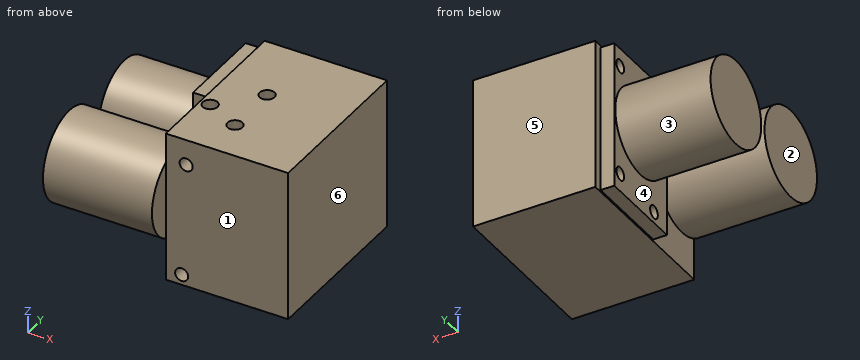
```python
from build123d import *

# Parameters (mm, degrees)
SKETCH2_W                        = 98.18
SKETCH2_H                        = 135.15
BOSS_EXTRUDE1_DEPTH              = 55.6
BOSS_EXTRUDE1_DEPTH_BACK         = 65.6
SKETCH3_R                        = 34.65
SKETCH3_R_2                      = 35.85
BOSS_EXTRUDE2_DEPTH              = 87.5
TAP_DRILL_FOR_M14X2_0_TAP1_D     = 12
TAP_DRILL_FOR_M14X2_0_TAP1_DEPTH = 19.56
TAP_DRILL_FOR_M14X2_0_TAP1_TIP   = 3.605163714
TAP_DRILL_FOR_M12X1_5_TAP2_D     = 10.5
TAP_DRILL_FOR_M12X1_5_TAP2_DEPTH = 19.56
TAP_DRILL_FOR_M12X1_5_TAP2_TIP   = 3.15451825
SKETCH8_W                        = 118.2
SKETCH8_H                        = 72
BOSS_EXTRUDE3_DEPTH              = 11
TAP_DRILL_FOR_M12X1_5_TAP3_D     = 10.5
TAP_DRILL_FOR_M12X1_5_TAP3_DEPTH = 19.56
TAP_DRILL_FOR_M12X1_5_TAP3_TIP   = 3.15451825


with BuildPart() as part:
    # Sketch2 → Boss-Extrude1 (new body, two sides)
    with BuildSketch(Plane.XY) as boss_extrude1_sk:
        Rectangle(SKETCH2_W, SKETCH2_H)
    extrude(amount=BOSS_EXTRUDE1_DEPTH)
    extrude(boss_extrude1_sk.sketch, amount=-BOSS_EXTRUDE1_DEPTH_BACK)

    # Sketch3 → Boss-Extrude2 (add)
    with BuildSketch(Plane.ZY.offset(49.09)):
        with Locations((0, 24.325)):
            Circle(SKETCH3_R)
        with Locations((0, -50.675)):
            Circle(SKETCH3_R_2)
    extrude(amount=BOSS_EXTRUDE2_DEPTH)

    # Tap Drill for M14x2.0 Tap1
    with Locations(Plane.XY.offset(55.6)):
        with Locations((-13.23, 9.825), (-13.23, -34.075), (-41.09, -20.575)):
            Hole(TAP_DRILL_FOR_M14X2_0_TAP1_D / 2, depth=TAP_DRILL_FOR_M14X2_0_TAP1_DEPTH)
            with Locations((0, 0, -(TAP_DRILL_FOR_M14X2_0_TAP1_DEPTH + TAP_DRILL_FOR_M14X2_0_TAP1_TIP / 2))):  # 118° drill point
                Cone(0, TAP_DRILL_FOR_M14X2_0_TAP1_D / 2, TAP_DRILL_FOR_M14X2_0_TAP1_TIP, mode=Mode.SUBTRACT)

    # Tap Drill for M12x1.5 Tap2
    with Locations(Plane(origin=(0, -67.575, 0), x_dir=(-1, 0, 0), z_dir=(0, -1, 0))):
        with Locations((32.79, -35.1), (36.39, 57.2)):
            Hole(TAP_DRILL_FOR_M12X1_5_TAP2_D / 2, depth=TAP_DRILL_FOR_M12X1_5_TAP2_DEPTH)
            with Locations((0, 0, -(TAP_DRILL_FOR_M12X1_5_TAP2_DEPTH + TAP_DRILL_FOR_M12X1_5_TAP2_TIP / 2))):  # 118° drill point
                Cone(0, TAP_DRILL_FOR_M12X1_5_TAP2_D / 2, TAP_DRILL_FOR_M12X1_5_TAP2_TIP, mode=Mode.SUBTRACT)

    # Sketch8 → Boss-Extrude3 (add)
    with BuildSketch(Plane.ZY.offset(49.09)):
        with Locations((-5, 24.325)):
            Rectangle(SKETCH8_W, SKETCH8_H)
    extrude(amount=BOSS_EXTRUDE3_DEPTH)

    # Tap Drill for M12x1.5 Tap3
    with Locations(Plane.ZY.offset(60.09)):
        with Locations((-49.6, 52.175), (-55.1, 6.075), (45.1, 6.075), (39.6, 52.175)):
            Hole(TAP_DRILL_FOR_M12X1_5_TAP3_D / 2, depth=TAP_DRILL_FOR_M12X1_5_TAP3_DEPTH)
            with Locations((0, 0, -(TAP_DRILL_FOR_M12X1_5_TAP3_DEPTH + TAP_DRILL_FOR_M12X1_5_TAP3_TIP / 2))):  # 118° drill point
                Cone(0, TAP_DRILL_FOR_M12X1_5_TAP3_D / 2, TAP_DRILL_FOR_M12X1_5_TAP3_TIP, mode=Mode.SUBTRACT)


solid = part.part
```
Source: CAD feature listing. Evaluate the final solid. Frame: model axes, mm. Face numbers are marked on the shaded views. A direction names the side the tool comes from. Give positions to 0.01 mm unless a question says otherwise; leave off trailing zeros. Loops run counter-clockwise (first coordinate to the right, second up) from the corner with the lowest first, then second, coordinate; pieces in that order, holes last. Notation, with made-up numbers: (59, 19.25) -> (105, 19.25) arc R15 cw to (105, 33.25) -> close; hole circle Ø3 at (2.25, 37.25). An arc over 180 degrees is marked (long way). Use a Markdown table: item, result. Add a question column.
(1) Section query B-B (x = -123). Output: boundary loops of the cut face in (y, z) (3 decimals).
(2) Pull-direction query (Y, two-part tool) for the marked faces 4, 5 and 6; classes: +Y half, -Y half, draft (parallel to the pull), parting line (faces both ways), or undercut.
(3) Ray query, line 1 (Z direction, x = -56, y = 48); line 2 (X direction, y = -58, z = 35); line 3 (Y direction, x = -54, z = -53.5) (3 decimals). Return the intervals inside material, ascending.
(4) Section query C-C (x = 14.5). Output: boundary loops of the cut face in (y, z) (3 decimals).
(5) Access query for the marked faces 1, 2 and 3. Directions: +Z, -Z, +X, -X, +Y, -Y. A direction counts if a zero-diameter tool reaches every point of the face in a straight line with its end or side. Return the directions, or none.
(6) First-contact query: pin 1 Ø2 at (y, z) = (-3, -42.5) entering from -X; pin 2 Ø6 at (x, y) = (-58, -66) entering from -Z; pin 3 Ø3.5 at (x, z) = (-57, -28) entering from +Y (3 decimals). Flat tips, straight axial feed; report the tip coordinate or a pass-through.
(7) Section query A-A (z = 0). Output: boundary loops of the cut face in (x, y) (3 decimals), then the cut area to 3 significant figures.
(8) Section query D-D (y = 37). Output: boundary loops of the cut face in (x, z), then the cut area to 3 significant figures.
Checked values:
| question | item | result |
|---|---|---|
| 1 | outline | circle Ø71.7 at (-50.675, 0); circle Ø69.3 at (24.325, 0) |
| 2 | face 4 | undercut |
| 2 | face 5 | +Y half |
| 2 | face 6 | draft |
| 3 | line 1 | -64.1 to -52.78, -46.42 to 36.42, 42.78 to 54.1 |
| 3 | line 2 | -136.59 to -38.04, -27.54 to 49.09 |
| 3 | line 3 | -11.675 to 1.075, 11.075 to 48.66, 55.69 to 60.325 |
| 4 | outline | (-67.575, -65.6) -> (67.575, -65.6) -> (67.575, 55.6) -> (-67.575, 55.6) -> close |
| 5 | face 1 | +Z, -Z, +X, -Y |
| 5 | face 2 | +Z, -Z, -X, +Y, -Y |
| 5 | face 3 | -X |
| 6 | pin 1 | x = -60.09 |
| 6 | pin 2 | z = -33.66 |
| 6 | pin 3 | y = 60.325 |
| 7 | outline | (-136.59, -86.525) -> (-49.09, -86.525) -> (-49.09, -67.575) -> (49.09, -67.575) -> (49.09, 67.575) -> (-49.09, 67.575) -> (-49.09, 60.325) -> (-60.09, 60.325) -> (-60.09, 58.975) -> (-136.59, 58.975) -> (-136.59, -10.325) -> (-60.09, -10.325) -> (-60.09, -11.675) -> (-49.09, -11.675) -> (-49.09, -14.825) -> (-136.59, -14.825) -> close |
| 7 | area | 25,600 mm^2 |
| 8 | outline | (-136.59, -32.25) -> (-60.09, -32.25) -> (-60.09, -64.1) -> (-49.09, -64.1) -> (-49.09, -65.6) -> (49.09, -65.6) -> (49.09, 55.6) -> (-49.09, 55.6) -> (-49.09, 54.1) -> (-60.09, 54.1) -> (-60.09, 32.25) -> (-136.59, 32.25) -> close |
| 8 | area | 18,100 mm^2 |
